Check sheet for the modelled part. Datum: model origin and axes. Units: mm. Face numbers are marked on the shaded views. A direction names the side the tool comes from. Round coordinates to 2 decimals unless told otherwise and drop trailing zeros. Order: outer loops, then holes, each group sorted by start corner. A loop starts at its lowest first (then second) coordinate and runs counter-clockwise, first axis right, second up.
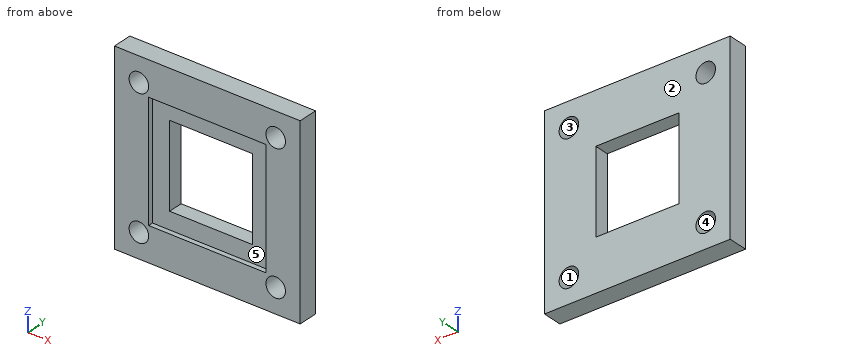
from build123d import *

# Parameters (mm, degrees)
SKETCH_W        = 38
SKETCH_H        = 38
SKETCH_R        = 2
PAD_DEPTH       = 4
SKETCH001_W     = 24
SKETCH001_H     = 24
POCKET_DEPTH    = 1
SKETCH002_W     = 17
SKETCH002_H     = 17
POCKET001_DEPTH = 3.001


with BuildPart() as part:
    # Sketch → Pad (new body)
    with BuildSketch(Plane.XZ):
        Rectangle(SKETCH_W, SKETCH_H)
        with Locations((-14, 14)):
            Circle(SKETCH_R, mode=Mode.SUBTRACT)
        with Locations((14, 14)):
            Circle(SKETCH_R, mode=Mode.SUBTRACT)
        with Locations((14, -14)):
            Circle(SKETCH_R, mode=Mode.SUBTRACT)
        with Locations((-14, -14)):
            Circle(SKETCH_R, mode=Mode.SUBTRACT)
    extrude(amount=PAD_DEPTH)

    # Sketch001 (on Face10 of Pad) → Pocket (cut)
    with BuildSketch(Plane.XZ.offset(4)):
        Rectangle(SKETCH001_W, SKETCH001_H)
    extrude(amount=-POCKET_DEPTH, mode=Mode.SUBTRACT)

    # Sketch002 (on Face15 of Pocket) → Pocket001 (cut, through all)
    with BuildSketch(Plane.XZ.offset(3)):
        Rectangle(SKETCH002_W, SKETCH002_H)
    extrude(amount=-POCKET001_DEPTH, mode=Mode.SUBTRACT)


solid = part.part
1) Gauge pin test, flat ends, axial feed: pin 1 (12 mm diameter, centred on x = -14.5, z = -7, fed in from +Y); pin 2 (10 mm diameter, centred on x = 1, z = 0.5, fed in from -Y). Record the tip position at first contact, or that the pin passes through.
2) Sectioned sample at D-D on z = 7. Record the cut outline in (x, y), and give its area (3 significant figures).
3) Scan lines: line 1 (Z direction, x = 14, y = -1.15); line 2 (X direction, y = -1.4, z = -7). Record each from-to range of solid material in increasing order.
4) Set-up check for the marked faces 4 and 5: record each of +Z, -Z, +X, -X, +Y, -Y from which the full face is reachable in a straight line by a thin tool's end or side.
5) Sectioned sample at A-A on x = 5.5. Record the cut outline in (y, z).
6) Sectioned sample at B-B on z = 14. Record the cut outline in (x, y), and give its area (3 significant figures).
7) Sectioned sample at C-C on y = -1. Record the cut outline in (x, z), and give its area (3 significant figures).
8) Draft check along X on the marked faces 1, 2 and 3. Enter one of: pulls with the +X half, pulls with the -X half, needs draft (parallel to the pull), parting line crosses it, or undercut.
Values found:
1. pin 1: stops at y = 0
1. pin 2: passes through
2. outline: (-19, -4) - (-12, -4) - (-12, -3) - (-8.5, -3) - (-8.5, 0) - (-19, 0) - close; (8.5, -3) - (12, -3) - (12, -4) - (19, -4) - (19, 0) - (8.5, 0) - close
2. area: 77.0 mm2
3. line 1: z = -19 to -16, -12 to 12, 16 to 19
3. line 2: x = -19 to -8.5, 8.5 to 19
4. face 4: +Y, -Y
4. face 5: -Y
5. outline: (-4, -19) - (0, -19) - (0, -8.5) - (-3, -8.5) - (-3, -12) - (-4, -12) - close; (-4, 12) - (-3, 12) - (-3, 8.5) - (0, 8.5) - (0, 19) - (-4, 19) - close
6. outline: (-19, -4) - (-16, -4) - (-16, 0) - (-19, 0) - close; (-12, -4) - (12, -4) - (12, 0) - (-12, 0) - close; (16, -4) - (19, -4) - (19, 0) - (16, 0) - close
6. area: 120 mm2
7. outline: (-19, -19) - (19, -19) - (19, 19) - (-19, 19) - close; hole circle Ø4 at (-14, -14); hole circle Ø4 at (-14, 14); hole (-8.5, -8.5) - (8.5, -8.5) - (8.5, 8.5) - (-8.5, 8.5) - close; hole circle Ø4 at (14, -14); hole circle Ø4 at (14, 14)
7. area: 1,100 mm2
8. face 1: undercut
8. face 2: needs draft
8. face 3: undercut
